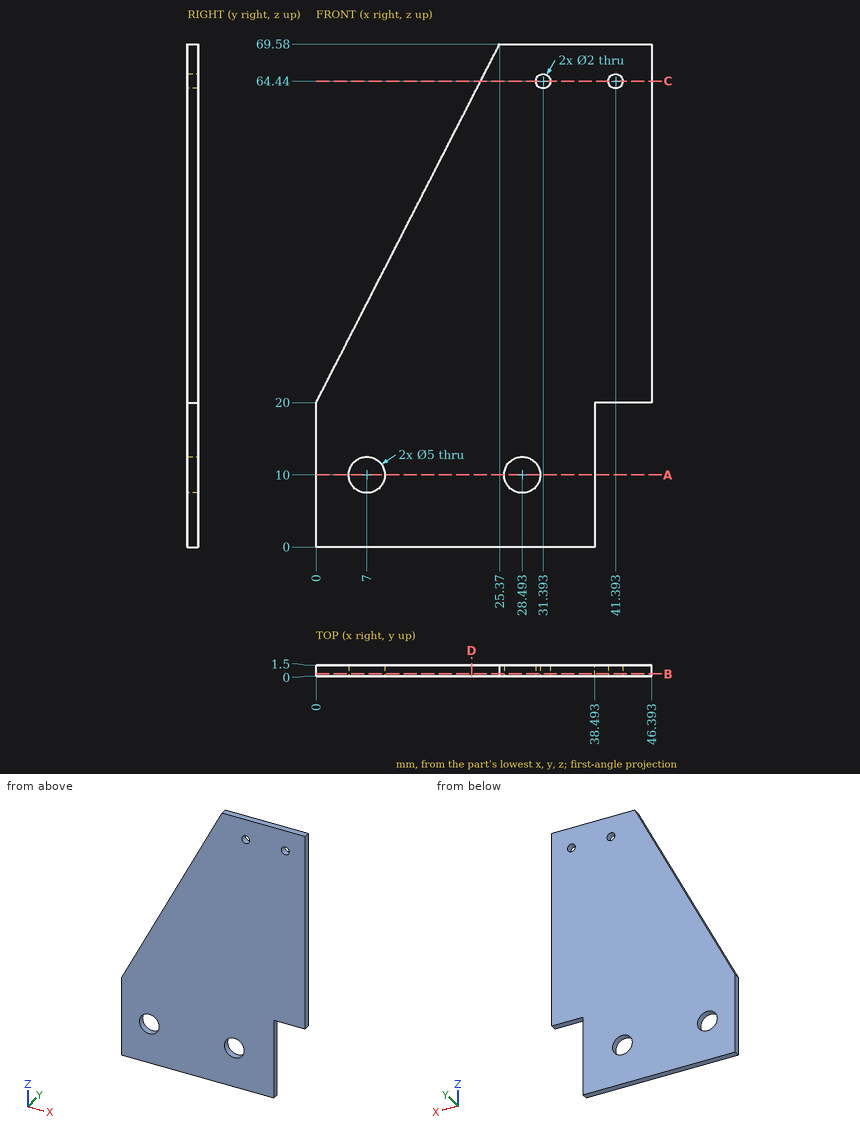
Check sheet for the drawn part. Datum: minimum x, y, z corner. Units: mm. Give positions to 0.01 mm unless a question says otherwise; leave off trailing zeros. Write each loop counter-clockwise with the first axis right and the second up, starting at its lowest first coordinate (ties: lowest second). Pieces come first, ordered by that corner, then holes.
(1) Cross-section at B-B (y = 0.3). Enter the section's corners in (x, z), plus the area to 3 significant figures.
(2) Gauge pin test, flat end, axial feed: pin 1 (1.2 mm diameter, centred on x = 41.39, z = 64.44, fed in from -Y). Record the tip position at first contact, or that the pin passes through.
(3) Material ranges on line 1 (X direction, y = 1, z = 10); line 2 (X direction, y = 0.85, z = 64.44); line 3 (Z direction, x = 30.5, y = 0.65), recorded low to high.
(4) Cross-section at D-D (x = 21.5). Enter the section's corners in (y, z).
(5) Cross-section at C-C (z = 64.44). Enter the section's corners in (x, y), plus the area to 3 significant figures.
(6) Cross-section at A-A (z = 10). Enter the section's corners in (x, y).
Worked out:
1. outline: (0, 0) - (38.49, 0) - (38.49, 20) - (46.39, 20) - (46.39, 69.58) - (25.37, 69.58) - (0, 20) - close; hole circle Ø5 at (7, 10); hole circle Ø5 at (28.49, 10); hole circle Ø2 at (31.39, 64.44); hole circle Ø2 at (41.39, 64.44)
1. area: 2,400 mm2
2. pin 1: passes through
3. line 1: x = 0 to 4.5, 9.5 to 25.99, 30.99 to 38.49
3. line 2: x = 22.74 to 30.39, 32.39 to 40.39, 42.39 to 46.39
3. line 3: z = 0 to 8.51, 11.49 to 63.99, 64.89 to 69.58
4. outline: (0, 0) - (1.5, 0) - (1.5, 62.02) - (0, 62.02) - close
5. outline: (22.74, 0) - (30.39, 0) - (30.39, 1.5) - (22.74, 1.5) - close; (32.39, 0) - (40.39, 0) - (40.39, 1.5) - (32.39, 1.5) - close; (42.39, 0) - (46.39, 0) - (46.39, 1.5) - (42.39, 1.5) - close
5. area: 29.5 mm2
6. outline: (0, 0) - (4.5, 0) - (4.5, 1.5) - (0, 1.5) - close; (9.5, 0) - (25.99, 0) - (25.99, 1.5) - (9.5, 1.5) - close; (30.99, 0) - (38.49, 0) - (38.49, 1.5) - (30.99, 1.5) - close
